Design review of the part built by this model. Coordinates are the model's own, in mm. A direction names the side the tool comes from. Give positions to 0.01 mm unless a question says otherwise; leave off trailing zeros. Loops run counter-clockwise (first coordinate to the right, second up) from the corner with the lowest first, then second, coordinate; pieces in that order, holes last. Notation, with made-up numbers: (-13, -33) -> (4, -33) arc R25 ccw to (4, -21) -> close; hole circle Ø9 at (82, 26). An arc over 180 degrees is marked (long way). Use a Markdown table: item, result. Add a question column.
1. Add section B-B (x = 46). State the section outline as (y, z) points (3 decimals), and give its area (3 significant figures).
2. To check wall thickness, follow line 1 (Z direction, x = 37.5, y = 1.65); line 2 (Y direction, x = -29.75, z = -24) (3 decimals); line 3 (Z direction, x = 28.5, y = 2.9). State the ranges of each line that lie inside material, in increasing order.
3. Add section D-D (z = -30). State the section outline as (x, y) points, and give its area (3 significant figures).
4. For pin 1 Ø0.9 at (y, z) = (2, -23.5) entering from -X; pin 2 Ø2.5 at (y, z) = (2, -22.5) entering from +X; pin 3 Ø0.9 at (y, z) = (2.5, 19) entering from +X, all flat-tipped, find the tip position at first contact; note any pin that passes through.
5. Add section C-C (y = 2.5). State the section outline as (x, z) points (3 decimals), and give its area (3 significant figures).
6. Add section A-A (z = 13). State the section outline as (x, y) points.
7. For faces 1 (the flat face through (22.5, 3, 20)), 2 (the flat face through (47.5, 2, -22)), 3 (the flat face through (47.5, 2, 23)), 4 (the flat face through (-22.5, 3, 13)), list the 3-axis set-ups (+Z, -Z, +X, -X, +Y, -Y) from which the entire face can be reached by the end or side of a thin tool; tool diameter is ignored.
8. Draft analysis for pull direction Y (two halves, no side actions). For faces 5 (the flat face through (2, 0, -1)), 6 (the flat face through (2, 5, -1)), 7 (the cylindrical face through (-35.2, 1.6, 11.9)), 8 (the flat face through (50, 2, -7.5)), state which applies: pulls with the +Y half, pulls with the -Y half, needs draft (parallel to the pull), parting line crosses it, or undercut.
```python
from build123d import *

# Parameters (mm, degrees)
SKETCH1_W           = 95
SKETCH1_H           = 75
BOSS_EXTRUDE1_DEPTH = 5
SKETCH3_W           = 15
SKETCH3_H           = 5
BOSS_EXTRUDE2_DEPTH = 5
SKETCH4_R           = 1.425
SKETCH4_R_2         = 1.422731811
CUT_EXTRUDE1_DEPTH  = 25
SKETCH5_R           = 1.425
CUT_EXTRUDE2_DEPTH  = 25
SKETCH6_R           = 1.425
CUT_EXTRUDE3_DEPTH  = 25


with BuildPart() as part:
    # Sketch1 → Boss-Extrude1 (new body)
    with BuildSketch(Plane(origin=(0, 0, 0), x_dir=(1, 0, 0), z_dir=(0, 1, 0))):
        Rectangle(SKETCH1_W, SKETCH1_H)
    extrude(amount=BOSS_EXTRUDE1_DEPTH)

    # Sketch3 → Boss-Extrude2 (add)
    with BuildSketch(Plane(origin=(47.5, 0, 0), x_dir=(0, 0, -1), z_dir=(1, 0, 0))):
        with Locations((0, 2.5)):
            Rectangle(SKETCH3_W, SKETCH3_H)
    extrude(amount=BOSS_EXTRUDE2_DEPTH)

    # Sketch4 → Cut-Extrude1 (cut)
    with BuildSketch(Plane.ZY.offset(47.5)):
        with Locations((-24, 2.5)):
            Circle(SKETCH4_R)
        with Locations((13, 2.5)):
            Circle(SKETCH4_R_2)
    extrude(amount=-CUT_EXTRUDE1_DEPTH, mode=Mode.SUBTRACT)

    # Sketch5 → Cut-Extrude2 (cut)
    with BuildSketch(Plane(origin=(47.5, 0, 0), x_dir=(0, 0, -1), z_dir=(1, 0, 0))):
        with Locations((-19.5, 2.5)):
            Circle(SKETCH5_R)
    extrude(amount=-CUT_EXTRUDE2_DEPTH, mode=Mode.SUBTRACT)

    # Sketch6 → Cut-Extrude3 (cut)
    with BuildSketch(Plane(origin=(47.5, 0, 0), x_dir=(0, 0, -1), z_dir=(1, 0, 0))):
        with Locations((25, 2.5)):
            Circle(SKETCH6_R)
    extrude(amount=-CUT_EXTRUDE3_DEPTH, mode=Mode.SUBTRACT)


solid = part.part
```
Taken from the geometry:
| question | item | result |
|---|---|---|
| 1 | outline | (0, -37.5) -> (5, -37.5) -> (5, 37.5) -> (0, 37.5) -> close; hole circle Ø2.85 at (2.5, -25); hole circle Ø2.85 at (2.5, 19.5) |
| 1 | area | 362 mm^2 |
| 2 | line 1 | z = -37.5 to -26.14, -23.86 to 18.36, 20.64 to 37.5 |
| 2 | line 2 | y = 0 to 1.075, 3.925 to 5 |
| 2 | line 3 | z = -37.5 to -26.37, -23.63 to 18.13, 20.87 to 37.5 |
| 3 | outline | (-47.5, 0) -> (47.5, 0) -> (47.5, 5) -> (-47.5, 5) -> close |
| 3 | area | 475 mm^2 |
| 4 | pin 1 | stops at x = -22.5 |
| 4 | pin 2 | stops at x = 47.5 |
| 4 | pin 3 | stops at x = 22.5 |
| 5 | outline | (-47.5, -37.5) -> (47.5, -37.5) -> (47.5, -26.425) -> (22.5, -26.425) -> (22.5, -23.575) -> (47.5, -23.575) -> (47.5, -7.5) -> (52.5, -7.5) -> (52.5, 7.5) -> (47.5, 7.5) -> (47.5, 18.075) -> (22.5, 18.075) -> (22.5, 20.925) -> (47.5, 20.925) -> (47.5, 37.5) -> (-47.5, 37.5) -> (-47.5, 14.423) -> (-22.5, 14.423) -> (-22.5, 11.577) -> (-47.5, 11.577) -> (-47.5, -22.575) -> (-22.5, -22.575) -> (-22.5, -25.425) -> (-47.5, -25.425) -> close |
| 5 | area | 6,920 mm^2 |
| 6 | outline | (-47.5, 0) -> (47.5, 0) -> (47.5, 5) -> (-47.5, 5) -> (-47.5, 3.92) -> (-22.5, 3.92) -> (-22.5, 1.08) -> (-47.5, 1.08) -> close |
| 7 | face 1 | +X |
| 7 | face 2 | -Z, +X, +Y, -Y |
| 7 | face 3 | +Z, +X, +Y, -Y |
| 7 | face 4 | -X |
| 8 | face 5 | pulls with the -Y half |
| 8 | face 6 | pulls with the +Y half |
| 8 | face 7 | undercut |
| 8 | face 8 | needs draft |
